from build123d import *

# Parameters (mm, degrees)
SKETCH1_R                = 6
BOSS_EXTRUDE1_DEPTH      = 98
BOSS_EXTRUDE2_START      = -42.489
SKETCH2_W                = 40
SKETCH2_H                = 13.022
BOSS_EXTRUDE2_DEPTH      = 13.022
BOSS_EXTRUDE3_DEPTH      = 30
BOSS_EXTRUDE3_DEPTH_BACK = 20
SKETCH4_W                = 13.022
SKETCH4_H                = 13.022
SKETCH6_W                = 10.902
SKETCH6_H                = 10.902
CUT_EXTRUDE1_DEPTH       = 60
BOSS_EXTRUDE4_START      = 10
SKETCH7_W                = 10.902
SKETCH7_H                = 10.902
BOSS_EXTRUDE4_DEPTH      = 20
SKETCH8_W                = 12
SKETCH8_H                = 25
BOSS_EXTRUDE5_DEPTH      = 30
SKETCH9_R                = 10
CUT_EXTRUDE2_DEPTH       = 100


with BuildPart() as part:
    # Sketch1 → Boss-Extrude1 (new body)
    with BuildSketch(Plane(origin=(0, 0, 0), x_dir=(1, 0, 0), z_dir=(0, 1, 0))):
        with Locations(Location((0, 0, 0), (0, 0, 270))):
            Circle(SKETCH1_R)
    extrude(amount=BOSS_EXTRUDE1_DEPTH)

    # Sketch2 → Boss-Extrude2 (add)
    with BuildSketch(Plane(origin=(0, 98, 0), x_dir=(1, 0, 0), z_dir=(0, 1, 0)).offset(BOSS_EXTRUDE2_START)):
        Rectangle(SKETCH2_W, SKETCH2_H)
    extrude(amount=-BOSS_EXTRUDE2_DEPTH)

    # Sketch4 → Boss-Extrude3 (add, two sides: drawn at the far end of the back side and taken through both)
    with BuildSketch(Plane.XY.offset(6.511).offset(-BOSS_EXTRUDE3_DEPTH_BACK)):
        with Locations((-26.511, 49)):
            Rectangle(SKETCH4_W, SKETCH4_H)
        with Locations((26.511, 49)):
            Rectangle(SKETCH4_W, SKETCH4_H)
    extrude(amount=BOSS_EXTRUDE3_DEPTH + BOSS_EXTRUDE3_DEPTH_BACK)

    # Sketch6 → Cut-Extrude1 (cut)
    with BuildSketch(Plane.XY.offset(36.511)):
        with Locations((-26.511, 49)):
            Rectangle(SKETCH6_W, SKETCH6_H)
        with Locations((26.511, 49)):
            Rectangle(SKETCH6_W, SKETCH6_H)
    extrude(amount=-CUT_EXTRUDE1_DEPTH, mode=Mode.SUBTRACT)

    # Sketch7 → Boss-Extrude4 (add)
    with BuildSketch(Plane.XY.offset(6.511).offset(BOSS_EXTRUDE4_START)):
        with Locations((-26.511, 49)):
            Rectangle(SKETCH7_W, SKETCH7_H)
        with Locations((26.511, 49)):
            Rectangle(SKETCH7_W, SKETCH7_H)
    extrude(amount=BOSS_EXTRUDE4_DEPTH)

    # Sketch8 → Boss-Extrude5 (add)
    with BuildSketch(Plane.XY.offset(36.511)):
        with Locations((-26.511, 49)):
            Rectangle(SKETCH8_W, SKETCH8_H)
        with Locations((26.511, 49)):
            Rectangle(SKETCH8_W, SKETCH8_H)
    extrude(amount=BOSS_EXTRUDE5_DEPTH)

    # Sketch9 → Cut-Extrude2 (cut)
    with BuildSketch(Plane.ZY.offset(32.511)):
        with Locations((51.511, 49)):
            Circle(SKETCH9_R)
    extrude(amount=-CUT_EXTRUDE2_DEPTH, mode=Mode.SUBTRACT)


solid = part.part
For this review, take the finished solid that the model builds, in its own axes (mm). A direction names the side the tool comes from. Round coordinates to 2 decimals unless told otherwise and drop trailing zeros. Loops run counter-clockwise (first coordinate to the right, second up) from the corner with the lowest first, then second, coordinate; pieces in that order, holes last. Notation, with made-up numbers: (0, 13.5) - (16, 13.5) arc R27 cw to (16, 47.5) - close; hole circle Ø11 at (-18, 58). An arc over 180 degrees is marked (long way). Use one line per item in the form item = value.
Item 1: Consider section A-A on z = 14.5. Write out the cut boundary in (x, y), then the cut area to 3 significant figures.
Answers:
outline = (-33.02, 42.49) - (-20, 42.49) - (-20, 55.51) - (-33.02, 55.51) - close; (20, 42.49) - (33.02, 42.49) - (33.02, 55.51) - (20, 55.51) - close; hole (-31.96, 43.55) - (-21.06, 43.55) - (-21.06, 54.45) - (-31.96, 54.45) - close; hole (21.06, 43.55) - (31.96, 43.55) - (31.96, 54.45) - (21.06, 54.45) - close
area = 101 mm^2
Item 2: For line 1 (X direction, y = 40, z = 63.5); line 2 (X direction, y = 48, z = 26); line 3 (Y direction, x = 22.5, z = -8), list the stretches that pass through material, from the lowest coordinate up.
Answers:
line_1 = -32.51 to -20.51, 20.51 to 32.51
line_2 = -33.02 to -20, 20 to 33.02
line_3 = 42.49 to 43.55, 54.45 to 55.51
Item 3: Consider section D-D on z = 33. Write out the cut boundary in (x, y).
Answers:
outline = (-33.02, 42.49) - (-20, 42.49) - (-20, 55.51) - (-33.02, 55.51) - close; (20, 42.49) - (33.02, 42.49) - (33.02, 55.51) - (20, 55.51) - close
Item 4: Mouldability with a two-part tool opening along X and no side actions: class faces 1 (the flat face through (-27, 40, 36.511)), 2 (the cylindrical face through (1.802, 20.947, 5.723)), 3 (the flat face through (26, 54.451, 2)) as +X half, -X half, draft (parallel to the pull), parting line (faces both ways), or undercut.
Answers:
face_1 = draft
face_2 = parting line
face_3 = undercut
Item 5: Clearance check with flat-ended pins moving along their axes: P1, Ø9.5, axis at x = -26.5, z = 58, coming from the +Y side; P2, Ø3.5, axis at x = -24, z = 4.5, coming from the -Y side; P3, Ø13, axis at x = -24, z = 58, coming from the -Y side. State where each tip first meets the part, or that it passes through.
Answers:
P1 = 61.5
P2 = 42.49
P3 = 36.5
Item 6: Consider section C-C on x = -26. Write out the cut boundary in (y, z).
Answers:
outline = (36.5, 36.51) - (42.49, 36.51) - (42.49, -13.49) - (43.55, -13.49) - (43.55, 16.51) - (54.45, 16.51) - (54.45, -13.49) - (55.51, -13.49) - (55.51, 36.51) - (61.5, 36.51) - (61.5, 66.51) - (36.5, 66.51) - close; hole circle Ø20 at (49, 51.51)
Item 7: Tool access review of faces 4 (the flat face through (-32.511, 49, 41)), 5 (the flat face through (26, 43.549, 2)), 6 (the flat face through (20, 49, 21)), 7 (the flat face through (-20, 49, -10)): name each direction out of +Z, -Z, +X, -X, +Y, -Y from which nothing blocks a thin tool from reaching the whole face with its end or side.
Answers:
face_4 = +Z, -X, +Y, -Y
face_5 = -Z
face_6 = +Z, +Y, -Y
face_7 = -Z, +Y, -Y
Item 8: Consider section B-B on z = 0. Write out the cut boundary in (x, y), then the cut area to 3 significant figures.
Answers:
outline = (-33.02, 42.49) - (-6, 42.49) - (-6, 0) - (6, 0) - (6, 42.49) - (33.02, 42.49) - (33.02, 55.51) - (6, 55.51) - (6, 98) - (-6, 98) - (-6, 55.51) - (-33.02, 55.51) - close; hole (-31.96, 43.55) - (-21.06, 43.55) - (-21.06, 54.45) - (-31.96, 54.45) - close; hole (21.06, 43.55) - (31.96, 43.55) - (31.96, 54.45) - (21.06, 54.45) - close
area = 1,640 mm^2
